```python
from build123d import *

# Parameters (mm, degrees)
PCB_DEPTH         = 1.6
HEADER_BODY_SK2_W = 2.54
HEADER_BODY_SK2_H = 35.52
HEADER_BODY_DEPTH = 2.5
HEADER_PINS_SK3_W = 0.64
HEADER_PINS_SK3_H = 33.72
HEADER_PINS_DEPTH = 5.8
STANDOFFS_SK4_R   = 1.765
STANDOFFS_DEPTH   = 2.5
M2_BORE_SK5_R     = 0.8
M2_BORE_DEPTH     = 3
USB_C_SK6_W       = 9.58
USB_C_SK6_H       = 7.71
USB_C_DEPTH       = 3.25
KEYS_SK7_W        = 4.56
KEYS_SK7_H        = 3.65
KEYS_DEPTH        = 1.81
CAM_FPC_SK8_W     = 17.2
CAM_FPC_SK8_H     = 5.69
CAM_FPC_DEPTH     = 2
BAT_CONN_SK9_W    = 7.65
BAT_CONN_SK9_H    = 5.2
BAT_CONN_DEPTH    = 3.4
TF_SLOT_SK10_W    = 11.4
TF_SLOT_SK10_H    = 5.5
TF_SLOT_DEPTH     = 2.7
ESP32_S3_SK11_W   = 5.12
ESP32_S3_SK11_H   = 14
ESP32_S3_DEPTH    = 1.8


with BuildPart() as part:
    # PCB_Sk1 → PCB (new body)
    with BuildSketch(Plane.XY.offset(-2)):
        with BuildLine():
            Line((-14.51, -25.81), (14.51, -25.81))
            ThreePointArc((14.51, -25.81), (16.631320344, -24.931320344), (17.51, -22.81))
            Line((17.51, -22.81), (17.51, 19.41))
            ThreePointArc((17.51, 19.41), (16.631320344, 21.531320344), (14.51, 22.41))
            Line((14.51, 22.41), (-14.51, 22.41))
            ThreePointArc((-14.51, 22.41), (-16.631320344, 21.531320344), (-17.51, 19.41))
            Line((-17.51, 19.41), (-17.51, -22.81))
            ThreePointArc((-17.51, -22.81), (-16.631320344, -24.931320344), (-14.51, -25.81))
        make_face()
    extrude(amount=-PCB_DEPTH)

    # Header_Body_Sk2 → Header_Body (add)
    with BuildSketch(Plane.XY.offset(-3.6)):
        with Locations((15.24, -1.7)):
            Rectangle(HEADER_BODY_SK2_W, HEADER_BODY_SK2_H)
        with Locations((-15.24, -1.7)):
            Rectangle(HEADER_BODY_SK2_W, HEADER_BODY_SK2_H)
    extrude(amount=-HEADER_BODY_DEPTH)

    # Header_Pins_Sk3 → Header_Pins (add)
    with BuildSketch(Plane.XY.offset(-6.1)):
        with Locations((15.24, -1.7)):
            Rectangle(HEADER_PINS_SK3_W, HEADER_PINS_SK3_H)
        with Locations((-15.24, -1.7)):
            Rectangle(HEADER_PINS_SK3_W, HEADER_PINS_SK3_H)
    extrude(amount=-HEADER_PINS_DEPTH)

    # Standoffs_Sk4 → Standoffs (add)
    with BuildSketch(Plane.XY.offset(-3.6)):
        with Locations((14.5, 19.4)):
            Circle(STANDOFFS_SK4_R)
        with Locations((-14.5, 19.4)):
            Circle(STANDOFFS_SK4_R)
        with Locations((14.5, -22.805)):
            Circle(STANDOFFS_SK4_R)
        with Locations((-14.5, -22.805)):
            Circle(STANDOFFS_SK4_R)
    extrude(amount=-STANDOFFS_DEPTH)

    # M2_Bore_Sk5 → M2_Bore (cut)
    with BuildSketch(Plane.XY.offset(-6.1)):
        with Locations((14.5, 19.4)):
            Circle(M2_BORE_SK5_R)
        with Locations((-14.5, 19.4)):
            Circle(M2_BORE_SK5_R)
        with Locations((14.5, -22.805)):
            Circle(M2_BORE_SK5_R)
        with Locations((-14.5, -22.805)):
            Circle(M2_BORE_SK5_R)
    extrude(amount=M2_BORE_DEPTH, mode=Mode.SUBTRACT)

    # USB_C_Sk6 → USB_C (add)
    with BuildSketch(Plane.XY.offset(-3.6)):
        with Locations((0, -23.135)):
            Rectangle(USB_C_SK6_W, USB_C_SK6_H)
    extrude(amount=-USB_C_DEPTH)

    # Keys_Sk7 → Keys (add)
    with BuildSketch(Plane.XY.offset(-3.6)):
        with Locations((9.475, -23.705)):
            Rectangle(KEYS_SK7_W, KEYS_SK7_H)
        with Locations((-9.45, -23.705)):
            Rectangle(KEYS_SK7_W, KEYS_SK7_H)
    extrude(amount=-KEYS_DEPTH)

    # Cam_FPC_Sk8 → Cam_FPC (add)
    with BuildSketch(Plane.XY.offset(-3.6)):
        with Locations((0, -12.475)):
            Rectangle(CAM_FPC_SK8_W, CAM_FPC_SK8_H)
    extrude(amount=-CAM_FPC_DEPTH)

    # Bat_Conn_Sk9 → Bat_Conn (add)
    with BuildSketch(Plane.XY.offset(-3.6)):
        with Locations((-9.095, -5.3)):
            Rectangle(BAT_CONN_SK9_W, BAT_CONN_SK9_H)
    extrude(amount=-BAT_CONN_DEPTH)

    # TF_Slot_Sk10 → TF_Slot (add)
    with BuildSketch(Plane.XY.offset(-3.6)):
        with Locations((-0.35, 4.25)):
            Rectangle(TF_SLOT_SK10_W, TF_SLOT_SK10_H)
    extrude(amount=-TF_SLOT_DEPTH)

    # ESP32_S3_Sk11 → ESP32_S3 (add)
    with BuildSketch(Plane.XY.offset(-3.6)):
        with Locations((9.56, 15)):
            Rectangle(ESP32_S3_SK11_W, ESP32_S3_SK11_H)
    extrude(amount=-ESP32_S3_DEPTH)


solid = part.part
```
Geometry check sheet. Reference: the model listing, model coordinates, mm. A direction names the side the tool comes from. Round coordinates to 2 decimals unless told otherwise and drop trailing zeros. Order: outer loops, then holes, each group sorted by start corner. A loop starts at its lowest first (then second) coordinate and runs counter-clockwise, first axis right, second up. Notation, with made-up numbers: M -30.5,19 L 23.5,19 A18 ccw 23.5,40 Z; hole C -25,-15 d8. An arc over 180 degrees is marked long. Write item = value, one per line.
Q1. Scan lines: line 1 (Y direction, x = 8, z = -4.5); line 2 (X direction, y = -4, z = -6.5); line 3 (Y direction, x = 14.5, z = -4.15) (3 decimals). Record each from-to range of solid material in increasing order.
Answer block:
line_1 = -25.53 to -21.88, -15.32 to -9.63, 8 to 22
line_2 = -15.56 to -14.92, -12.92 to -5.27, 14.92 to 15.56
line_3 = -24.57 to -23.605, -22.005 to -21.04, -19.46 to 16.06, 17.635 to 18.6, 20.2 to 21.165
Q2. Section check D-D (y = 4). Enter the section's corners in (x, z), plus the area to 3 significant figures.
Answer block:
outline = M -17.51,-3.6 L -16.51,-3.6 L -16.51,-6.1 L -15.56,-6.1 L -15.56,-11.9 L -14.92,-11.9 L -14.92,-6.1 L -13.97,-6.1 L -13.97,-3.6 L -6.05,-3.6 L -6.05,-6.3 L 5.35,-6.3 L 5.35,-3.6 L 13.97,-3.6 L 13.97,-6.1 L 14.92,-6.1 L 14.92,-11.9 L 15.56,-11.9 L 15.56,-6.1 L 16.51,-6.1 L 16.51,-3.6 L 17.51,-3.6 L 17.51,-2 L -17.51,-2 Z
area = 107 mm^2
Q3. Section check C-C (x = 6). Enter the section's corners in (y, z).
Answer block:
outline = M -25.81,-3.6 L -15.32,-3.6 L -15.32,-5.6 L -9.63,-5.6 L -9.63,-3.6 L 22.41,-3.6 L 22.41,-2 L -25.81,-2 Z
Q4. Set-up check for faces 1 (the flat face through (16.51, -2, -5)), 2 (the flat face through (-14.92, -2, -9)), 3 (the flat face through (-6.05, 4, -5)): record each of +Z, -Z, +X, -X, +Y, -Y from which the full face is reachable in a straight line by a thin tool's end or side.
Answer block:
face_1 = -Z, +X, +Y, -Y
face_2 = -Z, +Y, -Y
face_3 = -Z, +Y
Q5. Section check B-B (y = -1.5). Enter the section's corners in (x, z), plus the area to 3 significant figures.
Answer block:
outline = M -17.51,-3.6 L -16.51,-3.6 L -16.51,-6.1 L -15.56,-6.1 L -15.56,-11.9 L -14.92,-11.9 L -14.92,-6.1 L -13.97,-6.1 L -13.97,-3.6 L 13.97,-3.6 L 13.97,-6.1 L 14.92,-6.1 L 14.92,-11.9 L 15.56,-11.9 L 15.56,-6.1 L 16.51,-6.1 L 16.51,-3.6 L 17.51,-3.6 L 17.51,-2 L -17.51,-2 Z
area = 76.2 mm^2
Q6. Section check A-A (z = -10). Enter the section's corners in (x, y), plus the area to 3 significant figures.
Answer block:
outline = M -15.56,-18.56 L -14.92,-18.56 L -14.92,15.16 L -15.56,15.16 Z; M 14.92,-18.56 L 15.56,-18.56 L 15.56,15.16 L 14.92,15.16 Z
area = 43.2 mm^2
Q7. Depth check by flat-ended pin: pin 1 Ø3 at (x, z) = (-12, -6) entering from -Y; pin 2 Ø0.5 at (y, z) = (13.5, -4.5) entering from -X; pin 3 Ø4 at (x, y) = (-2, -24) entering from -Z. Enter the tip coordinate at first touch or a pass-through.
Answer block:
pin_1 = -25.53
pin_2 = -16.51
pin_3 = -6.85
Q8. Release check for a two-part mould opening along X. For faces 4 (the flat face through (0, 22.41, -3)), 5 (the flat face through (9, -21.88, -4)), 6 (the flat face through (-8.6, -13, -5)), 7 (the cylindrical face through (16.65, 21.51, -2.79)) record: released by +X, released by -X, zero draft, split by the parting line, or undercut.
Answer block:
face_4 = zero draft
face_5 = undercut
face_6 = undercut
face_7 = released by +X
